Geometry: final body of the model. Coordinates: model frame, mm. Give positions to 0.01 mm unless a question says otherwise; leave off trailing zeros. Write each loop counter-clockwise with the first axis right and the second up, starting at its lowest first coordinate (ties: lowest second). Pieces come first, ordered by that corner, then holes. Notation, with made-up numbers: M 62,20 L 96,20 A30 ccw 96,44 Z; hole C 61.5,20.25 d7. An arc over 180 degrees is marked long. Use a Markdown table: item, result. Add a question column.
1) Section C-C on x = -75.5. Return the cut outline in (y, z).
2) Section B-B on z = -54. Return the cut outline in (x, y).
3) Section D-D on z = -78. Return the cut outline in (x, y).
4) Line query: line 1 (Y direction, x = 121, z = 12); line 2 (Y direction, x = -105, z = -5.5); line 3 (X direction, y = 50.5, z = 12.5). Output: solid intervals per line, ascending.
5) Pin query (flat end, axial travel): pin 1 (6 mm diameter, centred on x = 29.5, y = 104.5, fed in from +Z); pin 2 (3.5 mm diameter, centred on y = 22.09, z = 12.5, fed in from +X) (3 decimals); pin 3 (4 mm diameter, centred on x = 97, y = 3.5, fed in from -Z); pin 4 (1 mm diameter, centred on y = 82.5, z = -69.5, fed in from -X). Return the tip coordinate at first contact, or that it passes through.
6) Section A-A on y = 75.5. Return the cut outline in (x, z).
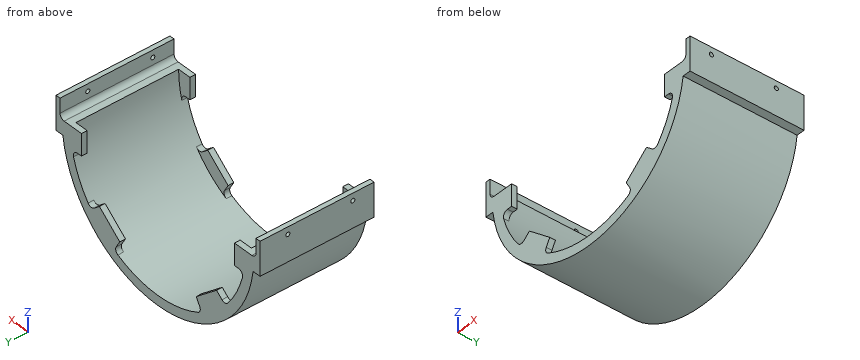
```python
from build123d import *

# Parameters (mm, degrees)
BOSS_EXTRUDE1_DEPTH    = 118.5
BOSS_EXTRUDE2_DEPTH    = 5.9
FILLET1_R              = 5
CUT_EXTRUDE1_START     = -5
CUT_EXTRUDE1_OUTLINE_R = 2.15
CUT_EXTRUDE1_DEPTH     = 5


# Read off the part's stored shape, not the designer's step: Cut-Extrude1
with BuildPart() as part:
    # Sketch1 → Boss-Extrude1 (new body)
    with BuildSketch(Plane(origin=(0, 0, 0), x_dir=(1, 0, 0), z_dir=(0, 1, 0))):
        with BuildLine():
            Line((-116.034477635, 15), (-124.5, 15))
            Line((-124.5, 15), (-124.5, -20))
            Line((-124.5, -20), (-119.5, -20))
            Line((-119.5, -20), (-119.5, 0))
            Line((-119.5, 0), (-107, 0))
            ThreePointArc((-107, 0), (0, 107), (107, 0))
            Line((107, 0), (119.5, 0))
            Line((119.5, 0), (119.5, -20))
            Line((119.5, -20), (124.5, -20))
            Line((124.5, -20), (124.5, 15))
            Line((124.5, 15), (116.034477635, 15))
            ThreePointArc((116.034477635, 15), (0, 117), (-116.034477635, 15))
        make_face()
    extrude(amount=BOSS_EXTRUDE1_DEPTH)

    # Sketch2 → Boss-Extrude2 (add)
    with BuildSketch(Plane(origin=(0, 118.5, 0), x_dir=(1, 0, 0), z_dir=(0, 1, 0))):
        Polygon((-113.25, 0), (-93.25, 0), (-93.25, 22.466274611), (-110.99922975, 22.466274611), align=None)
        Polygon((-86.754533183, 72.795696797), (-71.433644321, 59.939944603), (-46.625, 80.756868903), (-56.625, 98.077376979), align=None)
        Polygon((110.99922975, 22.466274611), (113.25, 0), (93.25, 0), (93.25, 22.466274611), align=None)
        Polygon((46.625, 80.756868903), (56.625, 98.077376979), (86.754533183, 72.795696797), (71.433644321, 59.939944603), align=None)
    boss_extrude2 = extrude(amount=-BOSS_EXTRUDE2_DEPTH)

    # Mirror1: Boss-Extrude2 across plane
    add(boss_extrude2.mirror(Plane.ZX.offset(59.25)))

    # Fillet1
    fillet1_edges = [part.edges().sort_by_distance(p)[0] for p in [
        (53.5, 115.55, -92.664718205),
        (81.966755414, 115.55, -68.778274236),
        (-104.614848397, 2.95, -22.466274611),
        (104.614848397, 2.95, -22.466274611),
        (-81.966755414, 2.95, -68.778274236),
        (-53.5, 2.95, -92.664718205),
        (81.966755414, 2.95, -68.778274236),
        (53.5, 2.95, -92.664718205),
        (119.5, 59.25, 0),
        (-119.5, 59.25, 0),
        (-104.614848397, 115.55, -22.466274611),
        (104.614848397, 115.55, -22.466274611),
        (-53.5, 115.55, -92.664718205),
        (-81.966755414, 115.55, -68.778274236),
    ]]
    fillet(fillet1_edges, radius=FILLET1_R)

    # Cut-Extrude1 outline → Cut-Extrude1 (cut)
    with BuildSketch(Plane.ZY.offset(-119.5).offset(CUT_EXTRUDE1_START)):
        with Locations((12.5, 22.085284338)):
            Circle(CUT_EXTRUDE1_OUTLINE_R)
        with Locations((12.5, 89.629742653)):
            Circle(CUT_EXTRUDE1_OUTLINE_R)
    cut_extrude1 = extrude(amount=CUT_EXTRUDE1_DEPTH, mode=Mode.SUBTRACT)

    # Mirror2: Cut-Extrude1 across plane
    add(cut_extrude1.mirror(Plane(origin=(0, 0, 0), x_dir=(0, 0, 1), z_dir=(1, 0, 0))), mode=Mode.SUBTRACT)


solid = part.part
```
Found:
| question | item | result |
|---|---|---|
| 1 | outline | M 0,-89.38 L 118.5,-89.38 L 118.5,-63.35 L 112.6,-63.35 L 112.6,-75.82 L 5.9,-75.82 L 5.9,-63.35 L 0,-63.35 Z |
| 2 | outline | M -103.79,0 L -92.37,0 L -92.37,118.5 L -103.79,118.5 Z; M 92.37,0 L 103.79,0 L 103.79,118.5 L 92.37,118.5 Z |
| 3 | outline | M -87.21,0 L -49.91,0 L -49.91,5.9 L -73.25,5.9 L -73.25,112.6 L -49.91,112.6 L -49.91,118.5 L -87.21,118.5 Z; M 49.91,0 L 87.21,0 L 87.21,118.5 L 49.91,118.5 L 49.91,112.6 L 73.25,112.6 L 73.25,5.9 L 49.91,5.9 Z |
| 4 | line 1 | 0 to 19.99, 24.18 to 87.54, 91.72 to 118.5 |
| 4 | line 2 | 0 to 5.9, 112.6 to 118.5 |
| 4 | line 3 | -124.5 to -119.5, 119.5 to 124.5 |
| 5 | pin 1 | z = -101.94 |
| 5 | pin 2 | through |
| 5 | pin 3 | z = -68.29 |
| 5 | pin 4 | x = -94.49 |
| 6 | outline | M -124.5,-15 L -116.03,-15 A117 ccw 116.03,-15 L 124.5,-15 L 124.5,20 L 119.5,20 L 119.5,5 A5 cw 114.5,0 L 107,0 A107 cw -107,0 L -114.5,0 A5 cw -119.5,5 L -119.5,20 L -124.5,20 Z |
